Here's how the part is built. I have some questions about the finished solid (model axes, mm). Coordinates: 2 decimals unless noted, no trailing zeros. Order: outer loops, then holes, each group sorted by start corner. A loop starts at its lowest first (then second) coordinate and runs counter-clockwise, first axis right, second up. Notation, with made-up numbers: (29, -1) - (53, -1) arc R27 ccw to (53, 15) - close; hole circle Ø8 at (-39, 30.25). An arc over 180 degrees is marked (long way). Answer in a Markdown table with one row per item. Add a question column.
Item 1: I want a section at B-B (y = 3). Please give me the cut outline in (x, z).
Item 2: Will these pins go through, and if not, where does the flat tip stop? pin 1 Ø0.9 at (x, z) = (2, -2) entering from -Y; pin 2 Ø1.5 at (y, z) = (-1, -2) entering from +X; pin 3 Ø0.9 at (y, z) = (2.5, -1.5) entering from -X.
Item 3: I want a section at C-C (x = 72). Please give me the cut outline in (y, z).
Item 4: If I drill on line 1 along Y through (x, z) = (90.5, -2.8); line 2 along X through (y, z) = (19, -0.95), over which ranges is the centre line in solid material (lowest first)? Write a range as from..to.
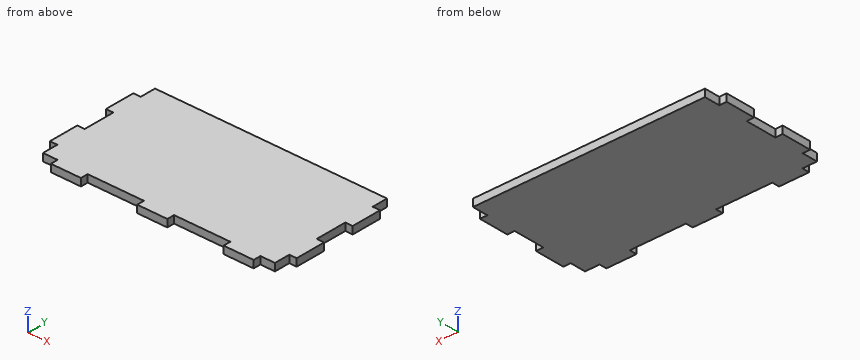
```python
from build123d import *

# Parameters (mm, degrees)
EXTRUDE_1_DEPTH = 3


with BuildPart() as part:
    # Эскиз1 → Бобышка-Вытянуть1 (new body)
    with BuildSketch(Plane.XY):
        Polygon((0, 0), (5.9, 0), (5.9, -3), (18.1, -3), (18.1, 0), (40.9, 0), (40.9, -3), (53.1, -3), (53.1, 0), (75.9, 0), (75.9, -3), (88.1, -3), (88.1, 0), (94, 0), (94, 6.4), (97, 6.4), (97, 18.6), (94, 18.6), (94, 31.4), (97, 31.4), (97, 43.6), (94, 43.6), (94, 50), (0, 50), (0, 43.6), (-3, 43.6), (-3, 31.4), (0, 31.4), (0, 18.6), (-3, 18.6), (-3, 6.4), (0, 6.4), align=None)
    extrude(amount=-EXTRUDE_1_DEPTH)


solid = part.part
```
Values follow:
| question | item | result |
|---|---|---|
| 1 | outline | (0, -3) - (94, -3) - (94, 0) - (0, 0) - close |
| 2 | pin 1 | stops at y = 0 |
| 2 | pin 2 | stops at x = 88.1 |
| 2 | pin 3 | stops at x = 0 |
| 3 | outline | (0, -3) - (50, -3) - (50, 0) - (0, 0) - close |
| 4 | line 1 | y = 0..50 |
| 4 | line 2 | x = 0..94 |
